from build123d import *

# Parameters (mm, degrees)
F0_R     = 1.778
F1_DEPTH = 1.5875


with BuildPart() as f1:
    # F0 (on Front) → F1 (new body, symmetric)
    with BuildSketch(Plane.XZ):
        Polygon((50.350482, -7.217964), (-44.899518, -7.217964), (-44.899518, -13.567964), (-41.724518, -13.567964), (-41.724518, -26.267964), (-44.899518, -26.267964), (-44.899518, -32.617964), (-13.149518, -32.617964), (-13.149518, -27.776089), (-15.340268, -27.776089), (-15.340268, -24.997964), (-13.149518, -24.997964), (-13.149518, -19.917964), (-9.593518, -19.917964), (-9.593518, -24.997964), (-7.402768, -24.997964), (-7.402768, -27.776089), (-9.593518, -27.776089), (-9.593518, -32.617964), (50.350482, -32.617964), align=None)
        with Locations((3.668914, -19.569241)):
            Circle(F0_R, mode=Mode.SUBTRACT)
        with Locations((37.650482, -19.569241)):
            Circle(F0_R, mode=Mode.SUBTRACT)
    extrude(amount=F1_DEPTH, both=True)


solid = f1.part
Work out the finished part from the listing and answer in its coordinate system (mm). A direction names the side the tool comes from. Round coordinates to 2 decimals unless told otherwise and drop trailing zeros. Write each loop counter-clockwise with the first axis right and the second up, starting at its lowest first coordinate (ties: lowest second). Pieces come first, ordered by that corner, then holes.
1) A cutting plane is placed at A-A (y = 0.3). Give the vertices of the cut face in (x, z), plus the area to 3 significant figures.
2) A cutting plane is placed at C-C (x = -11). Give the vertices of the cut face in (y, z), plus the area to 3 significant figures.
3) The mould has two halves that part along Z. Classify faces 6 (the flat face through (-41.725, 0, -20)), 7 (the flat face through (-13.15, 0, -30)), 8 (the flat face through (-14, 0, -27.776)), 9 (the flat face through (20, 0, -32.618)): pulls with the +Z half, pulls with the -Z half, needs draft (parallel to the pull), parting line crosses it, or undercut.
4) A cutting plane is placed at B-B (z = -18.75). Give the vertices of the cut face in (x, y).
5) A tool of negligible diameter and unlimited length cuts with its end or side. For faces 1 (the flat face through (-29, 0, -32.618)), 2 (the flat face through (-44.9, 0, -29)), 3 (the flat face through (-43, 0, -26.268)), 4 (the flat face through (-7.403, 0, -26)), 5 (the flat face through (-13.15, 0, -22)), from which of +Z, -Z, +X, -X, +Y, -Y can it reach the whole face along a straight path? Write none if from no direction.
6) Straight lines are drawn through the part: line 1 (X direction, y = 1.1, z = -29); line 2 (X direction, y = 1.3, z = -21.75); line 3 (X direction, y = -0.3, z = -20.5). For each, find the intervals that lie inside material, in ascending order.
7) A cutting plane is placed at D-D (z = -14.75). Give the vertices of the cut face in (x, y).
8) Given pin 1 Ø1 at (y, z) = (0, -23) entering from -X; pin 2 Ø3 at (x, z) = (37.65, -19.57) entering from +Y; pin 3 Ø1.6 at (x, y) = (-11.5, 0.5) entering from -Z, each flat-ended and moving along its own axis, determine where each tip first touches the part or whether it passes through.
Completed:
1. outline: (-44.9, -32.62) - (-13.15, -32.62) - (-13.15, -27.78) - (-15.34, -27.78) - (-15.34, -25) - (-13.15, -25) - (-13.15, -19.92) - (-9.59, -19.92) - (-9.59, -25) - (-7.4, -25) - (-7.4, -27.78) - (-9.59, -27.78) - (-9.59, -32.62) - (50.35, -32.62) - (50.35, -7.22) - (-44.9, -7.22) - (-44.9, -13.57) - (-41.72, -13.57) - (-41.72, -26.27) - (-44.9, -26.27) - close; hole circle Ø3.56 at (3.67, -19.57); hole circle Ø3.56 at (37.65, -19.57)
1. area: 2,300 mm2
2. outline: (-1.59, -19.92) - (1.59, -19.92) - (1.59, -7.22) - (-1.59, -7.22) - close
2. area: 40.3 mm2
3. face 6: undercut
3. face 7: needs draft
3. face 8: undercut
3. face 9: pulls with the -Z half
4. outline: (-41.72, -1.59) - (2.09, -1.59) - (2.09, 1.59) - (-41.72, 1.59) - close; (5.25, -1.59) - (36.07, -1.59) - (36.07, 1.59) - (5.25, 1.59) - close; (39.23, -1.59) - (50.35, -1.59) - (50.35, 1.59) - (39.23, 1.59) - close
5. face 1: -Z, +X, -X, +Y, -Y
5. face 2: +Z, -Z, -X, +Y, -Y
5. face 3: -X, +Y, -Y
5. face 4: +Y, -Y
5. face 5: -Z, +Y, -Y
6. line 1: x = -44.9 to -13.15, -9.59 to 50.35
6. line 2: x = -41.72 to -13.15, -9.59 to 50.35
6. line 3: x = -41.72 to -13.15, -9.59 to 2.15, 5.18 to 36.14, 39.17 to 50.35
7. outline: (-41.72, -1.59) - (50.35, -1.59) - (50.35, 1.59) - (-41.72, 1.59) - close
8. pin 1: stops at x = -41.72
8. pin 2: passes through
8. pin 3: stops at z = -19.92
